```python
from build123d import *

# Parameters (mm, degrees)
SKETCH1_W                   = 63.5
SKETCH1_H                   = 203.2
BOSS_EXTRUDE1_DEPTH         = 19.05
SKETCH2_R                   = 4.7625
CUT_EXTRUDE1_DEPTH          = 25.4
CUT_EXTRUDE2_DEPTH          = 9.525
SKETCH5_W                   = 38.1
SKETCH5_H                   = 8.128
CUT_EXTRUDE4_DEPTH          = 109.136603424
SKETCH6_W                   = 53.975
SKETCH6_H                   = 29.845
CUT_EXTRUDE5_DEPTH          = 2.159
F_1_4_20_TAPPED_HOLE1_D     = 5.1054
F_1_4_20_TAPPED_HOLE1_DEPTH = 19.05
F_1_4_20_TAPPED_HOLE1_TIP   = 1.533816902


with BuildPart() as part:
    # Sketch1 → Boss-Extrude1 (new body)
    with BuildSketch(Plane(origin=(0, 0, 0), x_dir=(1, 0, 0), z_dir=(0, 1, 0))):
        Rectangle(SKETCH1_W, SKETCH1_H)
    extrude(amount=BOSS_EXTRUDE1_DEPTH)

    # Sketch2 → Cut-Extrude1 (cut)
    with BuildSketch(Plane(origin=(0, 0, -101.6), x_dir=(-1, 0, 0), z_dir=(0, 0, -1))):
        Circle(SKETCH2_R)
    extrude(amount=-CUT_EXTRUDE1_DEPTH, mode=Mode.SUBTRACT)

    # Sketch3 → Cut-Extrude2 (cut)
    with BuildSketch(Plane(origin=(0, 0, 0), x_dir=(-1, 0, 0), z_dir=(0, -1, 0))):
        with BuildLine():
            Line((-20.6375, -96.8375), (20.6375, -96.8375))
            ThreePointArc((20.6375, -96.8375), (25.127628061, -94.977628061), (26.9875, -90.4875))
            Line((26.9875, -90.4875), (26.9875, 41.402))
            ThreePointArc((26.9875, 41.402), (25.127628061, 45.892128061), (20.6375, 47.752))
            Line((20.6375, 47.752), (-20.6375, 47.752))
            ThreePointArc((-20.6375, 47.752), (-25.127628061, 45.892128061), (-26.9875, 41.402))
            Line((-26.9875, 41.402), (-26.9875, -90.4875))
            ThreePointArc((-26.9875, -90.4875), (-25.127628061, -94.977628061), (-20.6375, -96.8375))
        make_face()
        with BuildLine():
            Line((-23.8125, 76.2), (23.8125, 76.2))
            ThreePointArc((23.8125, 76.2), (26.05756403, 75.27006403), (26.9875, 73.025))
            Line((26.9875, 73.025), (26.9875, 71.247))
            ThreePointArc((26.9875, 71.247), (26.05756403, 69.00193597), (23.8125, 68.072))
            Line((23.8125, 68.072), (-23.8125, 68.072))
            ThreePointArc((-23.8125, 68.072), (-26.05756403, 69.00193597), (-26.9875, 71.247))
            Line((-26.9875, 71.247), (-26.9875, 73.025))
            ThreePointArc((-26.9875, 73.025), (-26.05756403, 75.27006403), (-23.8125, 76.2))
        make_face()
    extrude(amount=-CUT_EXTRUDE2_DEPTH, mode=Mode.SUBTRACT)

    # Sketch5 → Cut-Extrude4 (cut, through all)
    with BuildSketch(Plane(origin=(0, 0, 0), x_dir=(1, 0, 0), z_dir=(0, 1, 0))):
        with Locations((0, 72.136)):
            Rectangle(SKETCH5_W, SKETCH5_H)
    extrude(amount=CUT_EXTRUDE4_DEPTH, mode=Mode.SUBTRACT)

    # Sketch6 → Cut-Extrude5 (cut)
    with BuildSketch(Plane(origin=(0, 0, 0), x_dir=(1, 0, 0), z_dir=(0, 1, 0))):
        with Locations((0, 56.3245)):
            Rectangle(SKETCH6_W, SKETCH6_H)
    extrude(amount=CUT_EXTRUDE5_DEPTH, mode=Mode.SUBTRACT)

    # 1/4-20 Tapped Hole1
    with Locations(Plane(origin=(-11.034450397, 19.05, 14.547513529), x_dir=(-1, 0, 0), z_dir=(0, 1, 0))):
        with Locations((-11.034450397, -52.647513529)):
            Hole(F_1_4_20_TAPPED_HOLE1_D / 2, depth=F_1_4_20_TAPPED_HOLE1_DEPTH)
            with Locations((0, 0, -(F_1_4_20_TAPPED_HOLE1_DEPTH + F_1_4_20_TAPPED_HOLE1_TIP / 2))):  # 118° drill point
                Cone(0, F_1_4_20_TAPPED_HOLE1_D / 2, F_1_4_20_TAPPED_HOLE1_TIP, mode=Mode.SUBTRACT)


solid = part.part
```
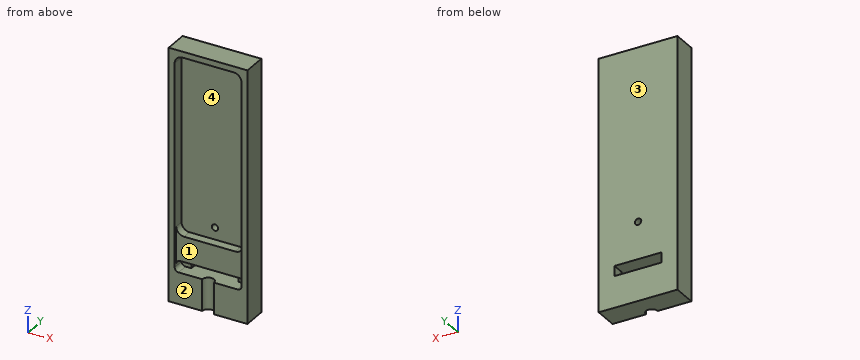
Work out the finished part from the listing and answer in its coordinate system (mm). Face numbers are marked on the shaded views. A direction names the side the tool comes from. Give positions to 0.01 mm unless a question says otherwise; leave off trailing zeros. Loops run counter-clockwise (first coordinate to the right, second up) from the corner with the lowest first, then second, coordinate; pieces in that order, holes last. Notation, with made-up numbers: (-7.5, -28) - (19.5, -28) arc R13 cw to (19.5, -21) - close; hole circle Ø5 at (14.5, 51.25). An arc over 180 degrees is marked (long way). Use CSV: the item, a comma, the result in double quotes. Start each with the question number.
(1) Find section C-C, the plane y = 15. Determine the outline of the cut face in (x, z).
(2) Find the intervals of material crossed by L1, parallel to Z at x = -10, y = 5.75; L2, parallel to Z at x = 0, y = 12.75; L3, parallel to Z at x = 11.5, y = 12.75, in increasing order.
(3) Each of these flat-tipped pins is pushed along its axis until it touches: pin 1 (1.5 mm diameter, centred on x = -24, z = 77, fed in from -Y) (3 decimals); pin 2 (3 mm diameter, centred on x = -1, z = -81, fed in from -Y); pin 3 (9 mm diameter, centred on x = -2.5, z = -51.5, fed in from -Y). Where does it stop, or does it pass through?
(4) A tool of negligible diameter and unlimited length cuts with its end or side. For the marked faces 3 and 4, from which of +Z, -Z, +X, -X, +Y, -Y can it reach the whole face along a straight path? Write none if from no direction.
(5) Find section A-A, the plane x = 0. Count the separate pieces of the cut face and the enclosed holes in it, plus the area to 3 significant figures.
(6) Determine the mould class of the marked faces 1 and 2 for opening direction X: released by +X, released by -X, zero draft, split by the parting line, or undercut.
Results found:
1,outline,"(-31.75, -101.6) - (31.75, -101.6) - (31.75, 101.6) - (-31.75, 101.6) - close; hole (-19.05, -76.2) - (19.05, -76.2) - (19.05, -68.07) - (-19.05, -68.07) - close; hole circle Ø5.11 at (0, -38.1)"
2,L1,"-101.6 to -76.2, -68.07 to -47.75, 96.84 to 101.6"
2,L2,"-101.6 to -76.2, -68.07 to -40.65, -35.55 to 101.6"
2,L3,"-101.6 to -76.2, -68.07 to 101.6"
3,pin 1,"y = 9.525"
3,pin 2,"y = 4.05"
3,pin 3,"y = 2.16"
4,face 3,"+Z, -Z, +X, -X, +Y"
4,face 4,"-Y"
5,separate pieces,"3"
5,enclosed holes,"0"
5,area,"2,130 mm^2"
6,face 1,"undercut"
6,face 2,"zero draft"
